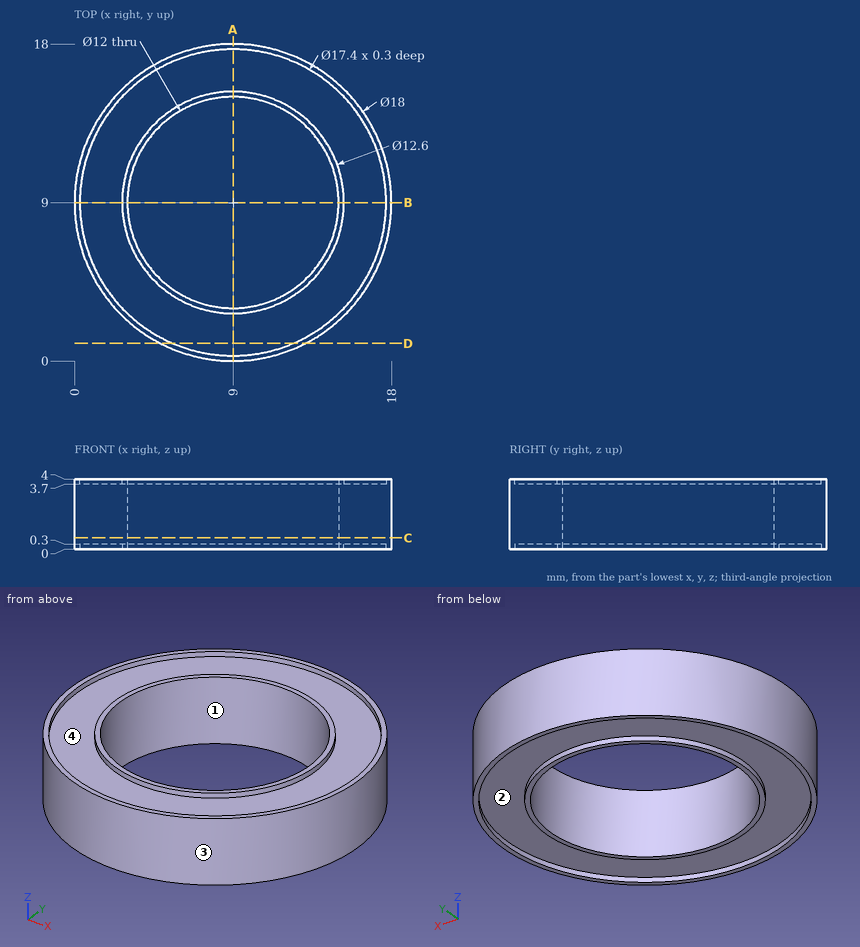
Design review of the part shown in the three views and the two pictorial views. Dimensions are in mm from the part's minimum x, y and z. A direction names the side the tool comes from. Give positions to 0.01 mm unless a question says otherwise; leave off trailing zeros. Order: outer loops, then holes, each group sorted by start corner. A loop starts at its lowest first (then second) coordinate and runs counter-clockwise, first axis right, second up. Notation, with made-up numbers: M 73,6 L 118,6 A10 cw 118,25 Z; hole C 2,19.25 d10. An arc over 180 degrees is marked long. Answer in a Markdown table with one row per item. Add a question column.
(1) Consider section C-C on z = 0.65. State the section outline as (x, y) points, and give its area (3 significant figures).
(2) For the marked faces 1 and 2, list the 3-axis set-ups (+Z, -Z, +X, -X, +Y, -Y) from which the entire face can be reached by the end or side of a thin tool; tool diameter is ignored.
(3) Mouldability with a two-part tool opening along X and no side actions: class the marked faces 3 and 4 as +X half, -X half, draft (parallel to the pull), parting line (faces both ways), or undercut.
(4) Consider section D-D on y = 1. State the section outline as (x, z) points, and give its area (3 significant figures).
(5) For pin 1 (8 mm diameter, centred on x = 3, y = 3.5, fed in from +Z); pin 2 (1 mm diameter, centred on y = 6.5, z = 1.5, fed in from -X); pin 3 (2 mm diameter, centred on x = 10.5, z = 1.5, fed in from +Y), all flat-tipped, find the tip position at first contact; note any pin that passes through.
(6) Consider section A-A on x = 9. State the section outline as (y, z) points, and give its area (3 significant figures).
(7) Wall thickness on probe 1 along Y at (x, z) = (9, 0.2); probe 2 along Y at (x, z) = (9, 2.15); probe 3 along X at (y, z) = (9.25, 2.05): over which ranges is each line inside the solid? List them lowest first. Write a range as [from, to].
Evaluation:
| question | item | result |
|---|---|---|
| 1 | outline | C 9,9 d18; hole C 9,9 d12 |
| 1 | area | 141 mm^2 |
| 2 | face 1 | +Z, -Z |
| 2 | face 2 | -Z |
| 3 | face 3 | parting line |
| 3 | face 4 | undercut |
| 4 | outline | M 4.88,0 L 5.58,0 L 5.58,0.3 L 12.42,0.3 L 12.42,0 L 13.12,0 L 13.12,4 L 12.42,4 L 12.42,3.7 L 5.58,3.7 L 5.58,4 L 4.88,4 Z |
| 4 | area | 28.9 mm^2 |
| 5 | pin 1 | stops at z = 4 |
| 5 | pin 2 | stops at x = 0.23 |
| 5 | pin 3 | stops at y = 17.99 |
| 6 | outline | M 0,0 L 0.3,0 L 0.3,0.3 L 2.7,0.3 L 2.7,0 L 3,0 L 3,4 L 2.7,4 L 2.7,3.7 L 0.3,3.7 L 0.3,4 L 0,4 Z; M 15,0 L 15.3,0 L 15.3,0.3 L 17.7,0.3 L 17.7,0 L 18,0 L 18,4 L 17.7,4 L 17.7,3.7 L 15.3,3.7 L 15.3,4 L 15,4 Z |
| 6 | area | 21.1 mm^2 |
| 7 | probe 1 | y = [0, 0.3], [2.7, 3], [15, 15.3], [17.7, 18] |
| 7 | probe 2 | y = [0, 3], [15, 18] |
| 7 | probe 3 | x = [0, 3.01], [14.99, 18] |
